The figure shows three views and two pictorial views of one solid part (mm, origin at its lowest corner). Answer the questions. Round coordinates to 2 decimals unless told otherwise and drop trailing zeros. Write each loop counter-clockwise with the first axis right and the second up, starting at its lowest first coordinate (ties: lowest second). Pieces come first, ordered by that corner, then holes. Notation, with made-up numbers: M -18.5,-12 L 2.5,-12 A25 cw 2.5,24 Z; hole C 73.5,73 d6. An arc over 180 degrees is marked long. Use one line per item in the form item = value. Start each with the question number.
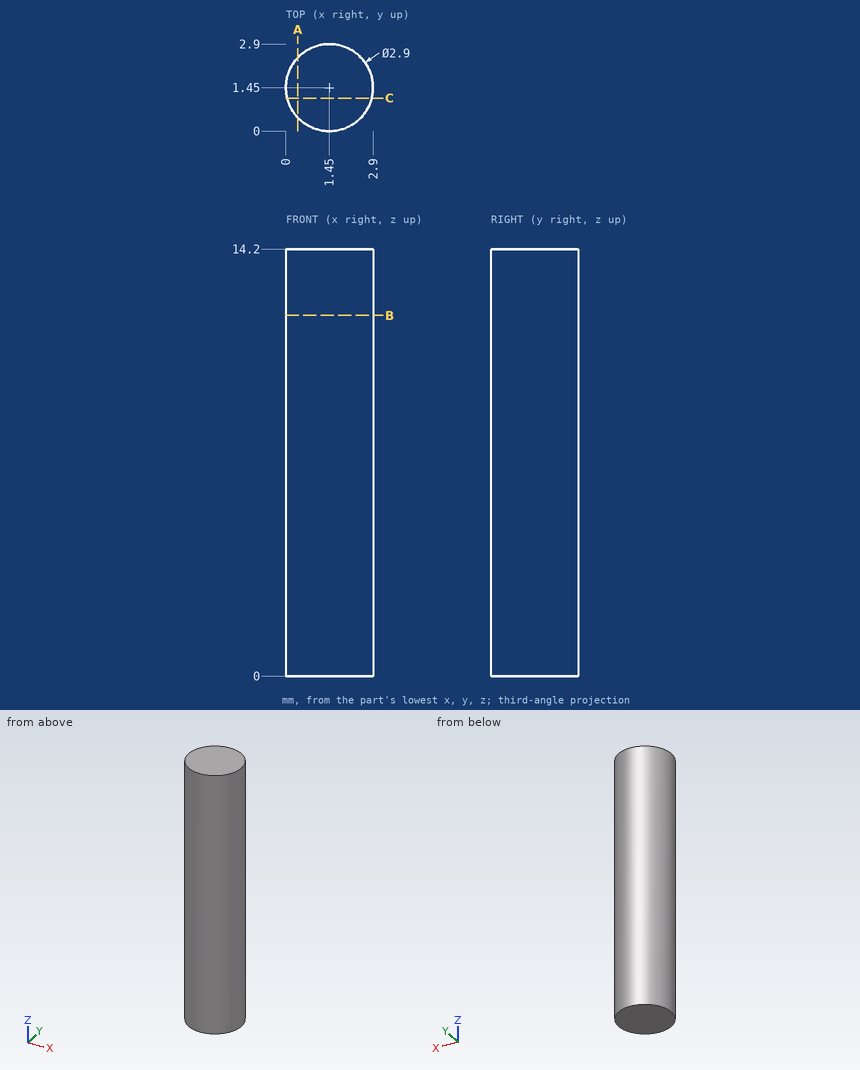
Q1. Find section A-A on x = 0.4. Write down the section's boundary in (y, z).
Q2. Straight lines are drawn through the part: line 1 (Y direction, x = 1.35, z = 5.5); line 2 (X direction, y = 1.8, z = 5.25); line 3 (Y direction, x = 2.6, z = 5.5). For each, find the intervals that lie inside material, in ascending order. Write a range as [from, to].
Q3. This flat-tipped pin is pushed along its axis until it touches: pin 1 Ø1 at (x, y) = (0.5, 2) entering from -Z. Where does it stop, or does it pass through?
Q4. Find section C-C on y = 1.1. Write down the section's boundary in (x, z).
Q5. Find section B-B on z = 12. Write down the section's boundary in (x, y), and give its area (3 significant figures).
Response:
q1.outline = M 0.45,0 L 2.45,0 L 2.45,14.2 L 0.45,14.2 Z
q2.line_1 = [0, 2.9]
q2.line_2 = [0.04, 2.86]
q2.line_3 = [0.57, 2.33]
q3.pin_1 = 0
q4.outline = M 0.04,0 L 2.86,0 L 2.86,14.2 L 0.04,14.2 Z
q5.outline = C 1.45,1.45 d2.9
q5.area = 6.61 mm²
